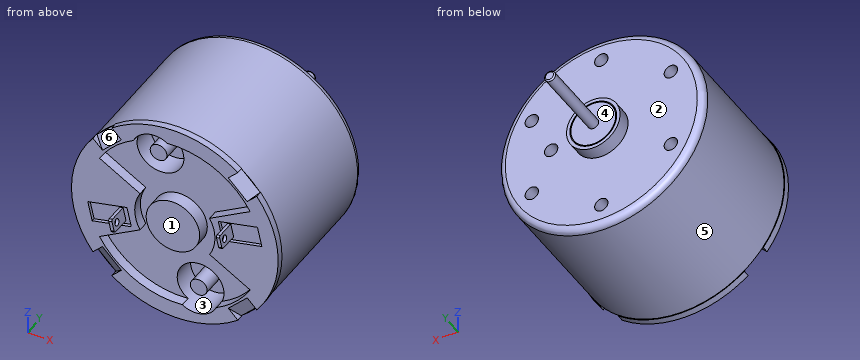
from build123d import *

# Parameters (mm, degrees)
ESBO_O1_R                  = 15.35
RESSALTO_EXTRUS_O1_DEPTH   = 21
ESBO_O2_R                  = 4
RESSALTO_EXTRUS_O2_DEPTH   = 2.1
ESBO_O3_R                  = 3.5
ESBO_O3_R_2                = 3.35
CORTE_EXTRUS_O1_DEPTH      = 1
ESBO_O4_R                  = 0.8
RESSALTO_EXTRUS_O3_DEPTH   = 11.5
FILETE1_R                  = 0.2
ESBO_O5_R                  = 1
CORTE_EXTRUS_O2_DEPTH      = 3
ESBO_O6_R                  = 1
CORTE_EXTRUS_O3_DEPTH      = 3
FILETE2_R                  = 1
ESBO_O7_R                  = 15.45
RESSALTO_EXTRUS_O4_DEPTH   = 1
CORTE_EXTRUS_O4_DEPTH      = 1.5
RESSALTO_EXTRUS_O5_START   = 2
ESBO_O9_R                  = 4
RESSALTO_EXTRUS_O5_DEPTH   = 2
CORTE_EXTRUS_O5_DEPTH      = 41.499567983
CORTE_EXTRUS_O5_DEPTH_BACK = 3.5
ESBO_O10_R                 = 3.5
ESBO_O11_R                 = 1.25
RESSALTO_EXTRUS_O6_DEPTH   = 4
CORTE_EXTRUS_O6_DEPTH      = 0.5
RESSALTO_EXTRUS_O7_DEPTH   = 3
ESBO_O15_R                 = 0.5
CORTE_EXTRUS_O7_DEPTH      = 46.395818321
FILETE3_R                  = 0.25
CORTE_EXTRUS_O8_DEPTH      = 1
CHANFRO1_SIZE              = 1.962610506
CHANFRO1_SIZE_2            = 1


with BuildPart() as part:
    # Esboço1 → Ressalto-extrusão1 (new body)
    with BuildSketch(Plane(origin=(0, 0, 0), x_dir=(1, 0, 0), z_dir=(0, 1, 0))):
        with Locations(Location((0, 0, 0), (0, 0, 90))):
            Circle(ESBO_O1_R)
    extrude(amount=RESSALTO_EXTRUS_O1_DEPTH)

    # Esboço2 → Ressalto-extrusão2 (add)
    with BuildSketch(Plane(origin=(0, 21, 0), x_dir=(1, 0, 0), z_dir=(0, 1, 0))):
        with Locations(Location((0, 0, 0), (0, 0, 270))):
            Circle(ESBO_O2_R)
    extrude(amount=RESSALTO_EXTRUS_O2_DEPTH)

    # Esboço3 → Corte-extrusão1 (cut)
    with BuildSketch(Plane(origin=(0, 23.1, 0), x_dir=(1, 0, 0), z_dir=(0, 1, 0))):
        with Locations(Location((0, 0, 0), (0, 0, 270))):
            Circle(ESBO_O3_R)
        with Locations(Location((0, 0, 0), (0, 0, 270))):
            Circle(ESBO_O3_R_2, mode=Mode.SUBTRACT)
    extrude(amount=-CORTE_EXTRUS_O1_DEPTH, mode=Mode.SUBTRACT)

    # Esboço4 → Ressalto-extrusão3 (add)
    with BuildSketch(Plane(origin=(0, 23.1, 0), x_dir=(1, 0, 0), z_dir=(0, 1, 0))):
        with Locations(Location((0, 0, 0), (0, 0, 270))):
            Circle(ESBO_O4_R)
    extrude(amount=RESSALTO_EXTRUS_O3_DEPTH)

    # Filete1
    filete1_edges = [part.edges().sort_by_distance(p)[0] for p in [
        (0, 34.6, -0.8),
    ]]
    fillet(filete1_edges, radius=FILETE1_R)

    # Esboço5 → Corte-extrusão2 (cut)
    with BuildSketch(Plane(origin=(0, 21, 0), x_dir=(1, 0, 0), z_dir=(0, 1, 0))):
        with Locations(Location((0, 12, 0), (0, 0, 270))):
            Circle(ESBO_O5_R)
        with Locations(Location((10.392304845, 6, 0), (0, 0, 270))):
            Circle(ESBO_O5_R)
        with Locations(Location((10.392304845, -6, 0), (0, 0, 270))):
            Circle(ESBO_O5_R)
        with Locations(Location((0, -12, 0), (0, 0, 270))):
            Circle(ESBO_O5_R)
        with Locations(Location((-10.392304845, -6, 0), (0, 0, 270))):
            Circle(ESBO_O5_R)
        with Locations(Location((-10.392304845, 6, 0), (0, 0, 270))):
            Circle(ESBO_O5_R)
    extrude(amount=-CORTE_EXTRUS_O2_DEPTH, mode=Mode.SUBTRACT)

    # Esboço6 → Corte-extrusão3 (cut)
    with BuildSketch(Plane(origin=(0, 21, 0), x_dir=(1, 0, 0), z_dir=(0, 1, 0))):
        with Locations(Location((7.5, 0, 0), (0, 0, 270))):
            Circle(ESBO_O6_R)
    extrude(amount=-CORTE_EXTRUS_O3_DEPTH, mode=Mode.SUBTRACT)

    # Filete2
    filete2_edges = [part.edges().sort_by_distance(p)[0] for p in [
        (0, 21, 15.35),
    ]]
    fillet(filete2_edges, radius=FILETE2_R)

    # Esboço7 → Ressalto-extrusão4 (add)
    with BuildSketch(Plane.XZ):
        with Locations(Location((0, 0, 0), (0, 0, 270))):
            Circle(ESBO_O7_R)
    extrude(amount=RESSALTO_EXTRUS_O4_DEPTH)

    # Esboço8 → Corte-extrusão4 (cut)
    with BuildSketch(Plane.XZ.offset(1)):
        with BuildLine():
            Line((-11.258330249, 6.5), (-5.196152423, 3))
            ThreePointArc((-5.196152423, 3), (-6, 0), (-5.196152423, -3))
            Line((-5.196152423, -3), (-11.258330249, -6.5))
            ThreePointArc((-11.258330249, -6.5), (0, -13), (11.258330249, -6.5))
            Line((11.258330249, -6.5), (5.196152423, -3))
            ThreePointArc((5.196152423, -3), (6, 0), (5.196152423, 3))
            Line((5.196152423, 3), (11.258330249, 6.5))
            ThreePointArc((11.258330249, 6.5), (0, 13), (-11.258330249, 6.5))
        make_face()
    extrude(amount=-CORTE_EXTRUS_O4_DEPTH, mode=Mode.SUBTRACT)

    # Esboço9 → Ressalto-extrusão5 (add)
    with BuildSketch(Plane.XZ.offset(-0.5).offset(RESSALTO_EXTRUS_O5_START)):
        with Locations(Location((0, 0, 0), (0, 0, 90))):
            Circle(ESBO_O9_R)
    extrude(amount=-RESSALTO_EXTRUS_O5_DEPTH)

    # Esboço10 → Corte-extrusão5 (cut, two sides: drawn at the far end of the back side and taken through both)
    with BuildSketch(Plane.XZ.offset(-0.5).offset(-CORTE_EXTRUS_O5_DEPTH_BACK)):
        with Locations(Location((-3, 10, 0), (0, 0, 57.495744103))):
            Circle(ESBO_O10_R)
        with Locations(Location((3, -10, 0), (0, 0, 335.902744365))):
            Circle(ESBO_O10_R)
    extrude(amount=CORTE_EXTRUS_O5_DEPTH + CORTE_EXTRUS_O5_DEPTH_BACK, mode=Mode.SUBTRACT)

    # Esboço11 → Ressalto-extrusão6 (add)
    with BuildSketch(Plane.XZ.offset(-4)):
        with Locations(Location((-3, 10, 0), (0, 0, 270))):
            Circle(ESBO_O11_R)
        with Locations(Location((3, -10, 0), (0, 0, 270))):
            Circle(ESBO_O11_R)
    extrude(amount=RESSALTO_EXTRUS_O6_DEPTH)

    # Esboço12 → Corte-extrusão6 (cut)
    with BuildSketch(Plane.XZ.offset(1)):
        Polygon((-6.498994273, -3.002178116), (-7.158511662, -0.075569701), (-13.011728492, -1.394604479), (-12.352211103, -4.321212894), align=None)
        Polygon((13.011728492, 1.394604479), (7.158511662, 0.075569701), (6.498994273, 3.002178116), (12.352211103, 4.321212894), align=None)
    extrude(amount=-CORTE_EXTRUS_O6_DEPTH, mode=Mode.SUBTRACT)

    # Esboço13 → Ressalto-extrusão7 (add)
    with BuildSketch(Plane.XZ.offset(0.5)):
        Polygon((-8.024128236, -0.7831769), (-7.584449976, -2.734249176), (-8.072218045, -2.844168741), (-8.511896305, -0.893096465), align=None)
        Polygon((8.511896305, 0.893096465), (8.024128236, 0.7831769), (7.584449976, 2.734249176), (8.072218045, 2.844168741), align=None)
    extrude(amount=RESSALTO_EXTRUS_O7_DEPTH)

    # Esboço15 → Corte-extrusão7 (cut, through all)
    with BuildSketch(Plane(origin=(-8.292057175, 0, -1.868632603), x_dir=(-0.21983912974654451, 0, 0.9755361382502865), z_dir=(-0.9755361382502864, 0, -0.2198391297465445))):
        with Locations((0, -2.5)):
            Circle(ESBO_O15_R)
    extrude(amount=-CORTE_EXTRUS_O7_DEPTH, mode=Mode.SUBTRACT)

    # Filete3
    filete3_edges = [part.edges().sort_by_distance(p)[0] for p in [
        (-8.26801227, -3.5, -0.838136682),
        (-7.828334011, -3.5, -2.789208959),
        (7.828334011, -3.5, 2.789208959),
        (8.26801227, -3.5, 0.838136682),
    ]]
    fillet(filete3_edges, radius=FILETE3_R)

    # Esboço16 → Corte-extrusão8 (cut)
    with BuildSketch(Plane.XZ.offset(1)):
        with BuildLine():
            Line((-12.270225276, 9.441798151), (-10.818733752, 7.990306627))
            Line((-10.818733752, 7.990306627), (-7.990306627, 10.818733752))
            Line((-7.990306627, 10.818733752), (-9.441798151, 12.270225276))
            ThreePointArc((-9.441798151, 12.270225276), (-10.947739051, 10.947739051), (-12.270225276, 9.441798151))
        make_face()
        with BuildLine():
            Line((7.990306627, 10.818733752), (9.441798151, 12.270225276))
            ThreePointArc((9.441798151, 12.270225276), (10.947739051, 10.947739051), (12.270225276, 9.441798151))
            Line((12.270225276, 9.441798151), (10.818733752, 7.990306627))
            Line((10.818733752, 7.990306627), (7.990306627, 10.818733752))
        make_face()
        with BuildLine():
            Line((12.270225276, -9.441798151), (10.818733752, -7.990306627))
            Line((10.818733752, -7.990306627), (7.990306627, -10.818733752))
            Line((7.990306627, -10.818733752), (9.441798151, -12.270225276))
            ThreePointArc((9.441798151, -12.270225276), (10.947739051, -10.947739051), (12.270225276, -9.441798151))
        make_face()
        with BuildLine():
            Line((-7.990306627, -10.818733752), (-9.441798151, -12.270225276))
            ThreePointArc((-9.441798151, -12.270225276), (-10.947739051, -10.947739051), (-12.270225276, -9.441798151))
            Line((-12.270225276, -9.441798151), (-10.818733752, -7.990306627))
            Line((-10.818733752, -7.990306627), (-7.990306627, -10.818733752))
        make_face()
    extrude(amount=-CORTE_EXTRUS_O8_DEPTH, mode=Mode.SUBTRACT)

    # Chanfro1
    # the kernel refuses this chamfer: 1.962610506, 1 mm, written as the material it adds along each edge
    with BuildSketch(Plane(origin=(10.818733752, 0, 7.990306627), x_dir=(0.7069981009602014, 0.017531984409911067, 0.7069981009601932), z_dir=(-0.7071067811865435, 0, 0.7071067811865517)), Plane(origin=(-10.818733752, 0, -7.990306627), x_dir=(-0.7069981009602017, 0.01753198440991109, -0.7069981009601931), z_dir=(0.7071067811865432, 0, -0.7071067811865519))) as chanfro1_piece_1:
        Polygon((CHANFRO1_SIZE * 0.999846302698, -CHANFRO1_SIZE * 0.0175319844055), (-CHANFRO1_SIZE_2 * 0.0175319844099, -CHANFRO1_SIZE_2 * 0.99984630295), (0, 0), align=None)
    extrude(amount=4)
    with BuildSketch(Plane(origin=(10.818733752, 0, -7.990306627), x_dir=(0.7069981009602014, 0.017531984409911067, -0.7069981009601932), z_dir=(-0.7071067811865435, 0, -0.7071067811865517)), Plane(origin=(-10.818733752, 0, 7.990306627), x_dir=(-0.7069981009602017, 0.01753198440991109, 0.7069981009601931), z_dir=(0.7071067811865432, 0, 0.7071067811865519))) as chanfro1_piece_2:
        Polygon((CHANFRO1_SIZE * 0.999846302698, CHANFRO1_SIZE * 0.0175319844055), (-CHANFRO1_SIZE_2 * 0.0175319844099, CHANFRO1_SIZE_2 * 0.99984630295), (0, 0), align=None)
    extrude(amount=4)


solid = part.part
Verification items for the finished model (mm, model axes). Face numbers are marked on the shaded views. A direction names the side the tool comes from. Coordinates: 2 decimals unless noted, no trailing zeros. Write each loop counter-clockwise with the first axis right and the second up, starting at its lowest first coordinate (ties: lowest second). Pieces come first, ordered by that corner, then holes. Notation, with made-up numbers: M 61,16.5 L 88,16.5 A21 ccw 88,48.5 Z; hole C 2.5,3 d1. An arc over 180 degrees is marked long. Use a Markdown table: item, result.
Q1. Sectioned sample at A-A, the plane y = 18.5. Record the boundary of the cut face in (x, z).
Reply:
| item | result |
|---|---|
| outline | C 0,0 d30.7; hole C -10.39,-6 d2; hole C -10.39,6 d2; hole C 0,-12 d2; hole C 0,12 d2; hole C 7.5,0 d2; hole C 10.39,-6 d2; hole C 10.39,6 d2 |
Q2. Sectioned sample at B-B, the plane y = 2.5. Record the boundary of the cut face in (x, z), plus the area to 3 significant figures.
Reply:
| item | result |
|---|---|
| outline | C 0,0 d30.7; C -3,10 d2.5; C 3,-10 d2.5; hole C -3,10 d7; hole C 3,-10 d7 |
| area | 673 mm² |
Q3. Sectioned sample at C-C, the plane y = 12. Record the boundary of the cut face in (x, z).
Reply:
| item | result |
|---|---|
| outline | C 0,0 d30.7 |
Q4. Draft check along X on the marked faces 4, 5 and 6. Enter one of: +X half, -X half, draft (parallel to the pull), parting line (faces both ways), or undercut.
Reply:
| item | result |
|---|---|
| face 4 | draft |
| face 5 | parting line |
| face 6 | undercut |
Q5. Go/stop test with flat-tipped pins: P1, Ø1.8, axis at x = -1, z = 13.5, coming from the +Y side; P2, Ø5.5, axis at x = -4, z = 8.5, coming from the -Y side; P3, Ø2.5, axis at x = 0, z = 12, coming from the -Y side. Record where each tip stops, or that it passes through.
Reply:
| item | result |
|---|---|
| P1 | stops at y = 21 |
| P2 | stops at y = 0 |
| P3 | stops at y = -1 |
Q6. Thickness scan on line 1 (X direction, y = 2.1, z = 10); line 2 (Y direction, x = 4, z = -5); line 3 (Y direction, x = 11.5, z = 6.5). Record the ranges inside material, lowest first.
Reply:
| item | result |
|---|---|
| line 1 | x = -11.65 to -6.5, -4.25 to -1.75, 0.5 to 11.65 |
| line 2 | y = 0.5 to 21 |
| line 3 | y = -1 to 21 |
Q7. Set-up check for the marked faces 1, 2 and 3: record each of +Z, -Z, +X, -X, +Y, -Y from which the full face is reachable in a straight line by a thin tool's end or side.
Reply:
| item | result |
|---|---|
| face 1 | +Z, -Z, -Y |
| face 2 | +Y |
| face 3 | -Y |
